from build123d import *

# Parameters (mm, degrees)
F0_W     = 4.7752
F0_H     = 869.95
F1_DEPTH = 1057.275
F2_W     = 4.7752
F2_H     = 869.95
F3_DEPTH = 31.75
F4_W     = 4.7752
F4_H     = 869.95
F5_DEPTH = 31.75
F6_W     = 1066.8
F6_H     = 4.7752
F7_DEPTH = 31.75
F8_W     = 1066.8
F8_H     = 4.7752
F9_DEPTH = 31.75


with BuildPart() as f1:
    # F0 (on Right) → F1 (new body)
    with BuildSketch(Plane.YZ):
        with Locations((-40.927166, 359.425986)):
            Rectangle(F0_W, F0_H)
    extrude(amount=F1_DEPTH)

    # F2 (on face) → F3 (join)
    with BuildSketch(Plane(origin=(0, -38.539566, 0), x_dir=(-1, 0, 0), z_dir=(0, 1, 0))):
        with Locations((-1054.8874, 359.425986)):
            Rectangle(F2_W, F2_H)
    extrude(amount=F3_DEPTH)

    # F4 (on face) → F5 (join)
    with BuildSketch(Plane(origin=(0, -38.539566, 0), x_dir=(-1, 0, 0), z_dir=(0, 1, 0))):
        with Locations((-2.3876, 359.425986)):
            Rectangle(F4_W, F4_H)
    extrude(amount=F5_DEPTH)

    # F6 (on face) → F7 (join)
    with BuildSketch(Plane(origin=(0, -38.539566, 0), x_dir=(-1, 0, 0), z_dir=(0, 1, 0))):
        with Locations((-533.4, -73.161414)):
            Rectangle(F6_W, F6_H)
    extrude(amount=F7_DEPTH)

    # F8 (on face) → F9 (join)
    with BuildSketch(Plane(origin=(0, -38.539566, 0), x_dir=(-1, 0, 0), z_dir=(0, 1, 0))):
        with Locations((-524.438678, 792.013386)):
            Rectangle(F8_W, F8_H)
    extrude(amount=F9_DEPTH)


solid = f1.part
Verification items for the finished model (mm, model axes). A direction names the side the tool comes from. Coordinates: 2 decimals unless noted, no trailing zeros. Write each loop counter-clockwise with the first axis right and the second up, starting at its lowest first coordinate (ties: lowest second). Pieces come first, ordered by that corner, then holes. Notation, with made-up numbers: (-8, -14.75) -> (50, -14.75) arc R27 cw to (50, 10.25) -> close; hole circle Ø8 at (67, 33.25). An arc over 180 degrees is marked (long way). One line per item, written item: value. Start each with the question number.
Q1. Cross-section at C-C on y = -27.5. Enter the section's corners in (x, z) (3 decimals), and give its area (3 significant figures).
Q2. Cross-section at B-B on x = 263. Enter the section's corners in (y, z), and give its area (3 significant figures).
Q3. Go/stop test with flat-tipped pins: P1, Ø2.5, axis at y = -21.5, z = 791, coming from the +X side; P2, Ø18.5, axis at y = -19, z = 485, coming from the +X side (3 decimals); P3, Ø2.5, axis at x = -4.5, y = -24.5, coming from the -Z side. Record where each tip stops, or that it passes through.
Q4. Mould release check, pull along X, two halves, no side actions. Record for faces 3 (the flat face through (536, -23, -70.774)), 4 (the flat face through (541, -25, -75.549)): pulls with the +X half, pulls with the -X half, needs draft (parallel to the pull), parting line crosses it, or undercut.
Q5. Cross-section at A-A on z = 342. Enter the section's corners in (x, y) (3 decimals).
Q6. Access from +Z, -Z, +X, -X, +Y, -Y to the whole of each face (thin tool, end or side, straight path). Record for faces 1 (the flat face through (4.775, -23, 353)), 2 (the flat face through (521, -43.315, 353)).
Q7. Thickness scan on L1, parallel to Z at x = 756.5, y = -32.5; L2, parallel to X at y = -27, z = 158.5 (3 decimals); L3, parallel to Y at x = 494, z = 20. Record the ranges inside material, lowest first. Write a range as from..to.
Checked values:
1. outline: (-8.961, 789.626) -> (0, 789.626) -> (0, -75.549) -> (1066.8, -75.549) -> (1066.8, -70.774) -> (1057.275, -70.774) -> (1057.275, 789.626) -> (1057.839, 789.626) -> (1057.839, 794.401) -> (-8.961, 794.401) -> close; hole (4.775, -70.774) -> (1052.5, -70.774) -> (1052.5, 789.626) -> (4.775, 789.626) -> close
1. area: 18,400 mm²
2. outline: (-43.31, -75.55) -> (-6.79, -75.55) -> (-6.79, -70.77) -> (-38.54, -70.77) -> (-38.54, 789.63) -> (-6.79, 789.63) -> (-6.79, 794.4) -> (-43.31, 794.4) -> close
2. area: 4,460 mm²
3. P1: stops at x = 1057.84
3. P2: stops at x = 1057.275
3. P3: stops at z = 789.63
4. face 3: undercut
4. face 4: needs draft
5. outline: (0, -43.315) -> (1057.275, -43.315) -> (1057.275, -6.79) -> (1052.5, -6.79) -> (1052.5, -38.54) -> (4.775, -38.54) -> (4.775, -6.79) -> (0, -6.79) -> close
6. face 1: +Y
6. face 2: +Z, -Z, +X, -X, -Y
7. L1: z = -75.55..-70.77, 789.63..794.4
7. L2: x = 0..4.775, 1052.5..1057.275
7. L3: y = -43.31..-38.54
